Part model, mm, in its own coordinate system. A direction names the side the tool comes from. Give positions to 0.01 mm unless a question says otherwise; leave off trailing zeros. Write each loop counter-clockwise with the first axis right and the second up, starting at its lowest first coordinate (ties: lowest second). Pieces come first, ordered by that corner, then holes. Notation, with made-up numbers: M 9,-10.75 L 59,-10.75 A20 ccw 59,11.25 Z; hole C 44,32.5 d8. An arc over 180 degrees is marked long. Use CSV: the item, a comma, the result in double quotes. Start each with the question number.
1. Drop flat-ended pins along their axis: pin 1 Ø3 at (x, y) = (-6.35, 6.35) entering from +Z; pin 2 Ø6 at (x, y) = (-0.5, 4.5) entering from -Z; pin 3 Ø4 at (x, y) = (1.5, 6.5) entering from -Z. Give the stop position or say it passes through.
2. Mould opens along Y. For faces 1 (the face through (-2, 1, -7.2)), 2 (the face through (0, 0, 2.29)), 3 (the face through (-7.271, 7.195, 1.129)), 4 (the face through (-0.867, 3.905, -0.993)) say: pulls with the +Y half, pulls with the -Y half, needs draft (parallel to the pull), parting line crosses it, or undercut.
3. 3-axis set-ups, long thin cutter, end or side, ignore diameter. For faces 5 (the face through (-2, -1, -8.4)), 6 (the face through (-4, 4, 2.29)), 7 (the face through (8.3, 8.27, 0.88)), 8 (the face through (-0.75, -0.03, -13.96)), 9 (the face through (0, 8.725, 1)): which of +Z, -Z, +X, -X, +Y, -Y reach the whole face in a straight line?
4. Band-saw the part on C-C, the plane z = 14. List the corners of the cut face in (x, y), then the cut area to 3 significant figures.
5. Band-saw the part on D-D, the plane z = -9. List the corners of the cut face in (x, y), then the cut area to 3 significant figures.
6. Band-saw the part on A-A, the plane y = -6.35. List the corners of the cut face in (x, z) (3 decimals), then the cut area to 3 significant figures.
7. Drill centre lines: line 1 along Y through (x, z) = (-6.35, 1.4) (3 decimals); line 2 along X through (y, z) = (0, -14.65); line 3 along Z through (x, y) = (-7, 0.5). Where is each one in solid material? Low to high. Write a range as from..to.
from build123d import *

# Parameters (mm, degrees)
F0_R      = 1.25
F1_DEPTH  = 2.29
F2_R      = 0.5
F3_R      = 5
F3_R_2    = 4.25
F4_DEPTH  = 15.88
F5_R      = 4
F6_DEPTH  = 1.5
F7_R      = 2.5
F8_DEPTH  = 10
F9_R      = 0.5
F12_R     = 1.25
F12_R_2   = 0.75
F13_DEPTH = 5


with BuildPart() as f1:
    # F0 (on Top) → F1 (new body)
    with BuildSketch(Plane.XY):
        with BuildLine():
            Line((-7.225, -8.725), (7.225, -8.725))
            ThreePointArc((7.225, -8.725), (8.28566, -8.28566), (8.725, -7.225))
            Line((8.725, -7.225), (8.725, 7.225))
            ThreePointArc((8.725, 7.225), (8.28566, 8.28566), (7.225, 8.725))
            Line((7.225, 8.725), (-7.225, 8.725))
            ThreePointArc((-7.225, 8.725), (-8.28566, 8.28566), (-8.725, 7.225))
            Line((-8.725, 7.225), (-8.725, -7.225))
            ThreePointArc((-8.725, -7.225), (-8.28566, -8.28566), (-7.225, -8.725))
        make_face()
        with Locations((-6.35, -6.35)):
            Circle(F0_R, mode=Mode.SUBTRACT)
        with Locations((6.35, -6.35)):
            Circle(F0_R, mode=Mode.SUBTRACT)
        with Locations((-6.35, 6.35)):
            Circle(F0_R, mode=Mode.SUBTRACT)
        with Locations((6.35, 6.35)):
            Circle(F0_R, mode=Mode.SUBTRACT)
    extrude(amount=F1_DEPTH)

    # F2
    f2_edges = [f1.edges().sort_by_distance(p)[0] for p in [
        (0, -8.725, 2.29),
    ]]
    fillet(f2_edges, radius=F2_R)

    # F3 (on face) → F4 (join)
    with BuildSketch(Plane.XY.offset(2.29)):
        Circle(F3_R)
        Circle(F3_R_2, mode=Mode.SUBTRACT)
    extrude(amount=F4_DEPTH)

    # F5 (on face) → F6 (join)
    with BuildSketch(Plane(origin=(0, 0, 0), x_dir=(1, 0, 0), z_dir=(0, 0, -1))):
        Circle(F5_R)
    extrude(amount=F6_DEPTH)

    # F7 (on face) → F8 (join)
    with BuildSketch(Plane(origin=(0, 0, -1.5), x_dir=(1, 0, 0), z_dir=(0, 0, -1))):
        Circle(F7_R)
    extrude(amount=F8_DEPTH)

    # F9
    f9_edges = [f1.edges().sort_by_distance(p)[0] for p in [
        (-4, 0, 0),
        (-2.5, 0, -11.5),
    ]]
    fillet(f9_edges, radius=F9_R)

    # F10 (on Right) → F11 (revolve, cut)
    with BuildSketch(Plane.YZ):
        Polygon((-2, -5), (-2, -4), (-6, -4), (-6, -9.4), (-2, -9.4), (-2, -8.4), (-3.5, -8.4), (-3.5, -7.2), (-2, -7.2), (-2, -6.2), (-3.5, -6.2), (-3.5, -5), align=None)
    revolve(axis=Axis((0, 0, -7.479729), (0, 0, -1)), mode=Mode.SUBTRACT)

    # F12 (on face) → F13 (join)
    with BuildSketch(Plane(origin=(0, 0, -11.5), x_dir=(1, 0, 0), z_dir=(0, 0, -1))):
        Circle(F12_R)
        Circle(F12_R_2, mode=Mode.SUBTRACT)
    extrude(amount=F13_DEPTH)


solid = f1.part
Output:
1,pin 1,"stops at z = 2.29"
1,pin 2,"stops at z = -11.5"
1,pin 3,"stops at z = 0"
2,face 1,"needs draft"
2,face 2,"undercut"
2,face 3,"undercut"
2,face 4,"parting line crosses it"
3,face 5,"none"
3,face 6,"+Z"
3,face 7,"+Z, -Z, +X, +Y"
3,face 8,"-Z"
3,face 9,"+Z, -Z, +X, -X, +Y"
4,outline,"C 0,0 d10; hole C 0,0 d8.5"
4,area,"21.8 mm²"
5,outline,"C 0,0 d4"
5,area,"12.6 mm²"
6,outline,"M -8.725,0 L -7.6,0 L -7.6,2.29 L -8.225,2.29 A0.5 ccw -8.725,1.79 Z; M -5.1,0 L 5.1,0 L 5.1,2.29 L -5.1,2.29 Z; M 7.6,0 L 8.725,0 L 8.725,1.79 A0.5 ccw 8.225,2.29 L 7.6,2.29 Z"
6,area,"28.4 mm²"
7,line 1,"y = -8.725..-7.6, -5.1..5.1, 7.6..8.725"
7,line 2,"x = -1.25..-0.75, 0.75..1.25"
7,line 3,"z = 0..2.29"
